```python
from build123d import *

# Parameters (mm, degrees)
SKETCH1_W            = 32
SKETCH1_H            = 26.941935484
SKETCH1_R            = 4
BOSS_EXTRUDE1_DEPTH  = 10
SKETCH2_W            = 10
SKETCH2_H            = 26.941935484
BOSS_EXTRUDE2_DEPTH  = 8
BOSS_EXTRUDE3_REACH  = 61.413
M5_CLEARANCE_HOLE1_D = 5.8
SKETCH6_W            = 52
SKETCH6_H            = 44.941935484
SKETCH6_R            = 4
BOSS_EXTRUDE4_DEPTH  = 6
M5_CLEARANCE_HOLE2_D = 5.8


with BuildPart() as part:
    # Sketch1 → Boss-Extrude1 (new body)
    with BuildSketch(Plane(origin=(0, 0, 0), x_dir=(1, 0, 0), z_dir=(0, 1, 0))):
        with Locations((16, 13.470967742)):
            Rectangle(SKETCH1_W, SKETCH1_H)
        with Locations(Location((16, 13.7, 0), (0, 0, 270))):
            Circle(SKETCH1_R, mode=Mode.SUBTRACT)
    extrude(amount=BOSS_EXTRUDE1_DEPTH)

    # Sketch2 → Boss-Extrude2 (add)
    with BuildSketch(Plane(origin=(0, 10, 0), x_dir=(1, 0, 0), z_dir=(0, 1, 0))):
        with Locations((-5, 13.470967742)):
            Rectangle(SKETCH2_W, SKETCH2_H)
        with Locations((37, 13.470967742)):
            Rectangle(SKETCH2_W, SKETCH2_H)
    extrude(amount=-BOSS_EXTRUDE2_DEPTH)

    # Boss-Extrude3: up to this face of the body (flat: up to its plane)
    boss_extrude3_end = Plane(part.part.faces().sort_by_distance((42, 6, -13.470967742))[0])
    # Sketch3 → Boss-Extrude3 (add, up to the picked face)
    with BuildSketch(Plane.ZY.offset(10), mode=Mode.PRIVATE) as boss_extrude3_sk1:
        Polygon((0, 0), (8, -8), (18, -8), (18, 10), (0, 10), align=None)
    boss_extrude3_tool1 = split(extrude(boss_extrude3_sk1.sketch, amount=-BOSS_EXTRUDE3_REACH, mode=Mode.PRIVATE), bisect_by=boss_extrude3_end, keep=Keep.BOTH, mode=Mode.PRIVATE)
    add(boss_extrude3_tool1.solids().sort_by(Axis((-10, 1.694064, 9.694064), (1, 0, 0)))[0])

    # M5 Clearance Hole1 (through all)
    with Locations(Plane(origin=(0, 0, -26.941935484), x_dir=(-1, 0, 0), z_dir=(0, 0, -1))):
        with Locations((-28, 6), (-4, 6)):
            Hole(M5_CLEARANCE_HOLE1_D / 2)

    # Sketch6 → Boss-Extrude4 (add)
    with BuildSketch(Plane(origin=(0, 10, 0), x_dir=(1, 0, 0), z_dir=(0, 1, 0))):
        with Locations((16, 4.470967742)):
            Rectangle(SKETCH6_W, SKETCH6_H)
        with Locations(Location((16, 13.7, 0), (0, 0, 270))):
            Circle(SKETCH6_R, mode=Mode.SUBTRACT)
    extrude(amount=BOSS_EXTRUDE4_DEPTH)

    # M5 Clearance Hole2 (through all)
    with Locations(Plane(origin=(0, 16, 0), x_dir=(1, 0, 0), z_dir=(0, 1, 0))):
        with Locations((37.04456925, 18.051391355), (36.92194463, 5.790370874), (-4.953330413, 18.47141973), (-5.075955034, 6.210399249)):
            Hole(M5_CLEARANCE_HOLE2_D / 2)


solid = part.part
```
Can you work these out from the model? Positions are in its coordinate system, mm. A direction names the side the tool comes from. Give positions to 0.01 mm unless a question says otherwise; leave off trailing zeros. Write each loop counter-clockwise with the first axis right and the second up, starting at its lowest first coordinate (ties: lowest second). Pieces come first, ordered by that corner, then holes. Notation, with made-up numbers: (-23.5, 72) - (-16.5, 72) arc R26 cw to (-16.5, 109) - close; hole circle Ø7 at (-16, 40). An arc over 180 degrees is marked (long way). Write item = value, one per line. Start each with the question number.
1. Imagine slicing it at B-B (z = -13.7). Please give me the cut outline in (x, y), and give its area (3 significant figures).
2. Imagine slicing it at D-D (y = 6). Please give me the cut outline in (x, z), and give its area (3 significant figures).
3. On a 3-axis mill with a long thin cutter (end or side, diameter ignored), from which of +Z, -Z, +X, -X, +Y, -Y can I reach the whole of each face in a straight line? I mean faces 1 (the face through (19.3, 0, -10.7)), 2 (the face through (32, 1, -13)), 3 (the face through (0, 1, -13)). Say none if no direction works.
4. For pin 1 (13.5 mm diameter, centred on x = 20, z = -14.5, fed in from -Y); pin 2 (1.6 mm diameter, centred on x = 38.5, y = 1, fed in from -Z); pin 3 (3.5 mm diameter, centred on x = 4, y = 6, fed in from -Z); pin 4 (0.6 mm diameter, centred on y = 1, z = -14.5, fed in from -X), each with a flat end and sliding along its axis, tell me the tip position at first contact or that it passes through.
5. Thinking about a two-plate mould opening in Z: for faces 4 (the face through (37, 1, 0)), 5 (the face through (37, 2, -14)), 6 (the face through (-2.65, 8.9, -16.71)), which applies, released by +Z, released by -Z, zero draft, split by the parting line, or undercut?
6. Imagine slicing it at C-C (x = 28). Please give me the cut outline in (y, z), and give its area (3 significant figures).
7. Please list where these lines run through material, in increasing order: line 1 (X direction, y = 4.75, z = -2); line 2 (Z direction, x = 36, y = 13); line 3 (Y direction, x = 4, z = -15.5).
8. Imagine slicing it at A-A (y = 0.75). Please give me the cut outline in (x, z), and give its area (3 significant figures).
Worked answers:
q1.outline = (-10, 2) - (0, 2) - (0, 0) - (12, 0) - (12, 16) - (-10, 16) - close; (20, 0) - (32, 0) - (32, 2) - (42, 2) - (42, 16) - (20, 16) - close; hole circle Ø5.8 at (4, 6); hole circle Ø5.8 at (28, 6)
q1.area = 611 mm2
q2.outline = (-10, -26.94) - (1.1, -26.94) - (1.1, 18) - (-10, 18) - close; (6.9, -26.94) - (25.1, -26.94) - (25.1, 18) - (6.9, 18) - close; (30.9, -26.94) - (42, -26.94) - (42, 18) - (30.9, 18) - close; hole circle Ø5.8 at (-5.08, -6.21); hole circle Ø5.8 at (-4.95, -18.47); hole circle Ø8 at (16, -13.7); hole circle Ø5.8 at (36.92, -5.79); hole circle Ø5.8 at (37.04, -18.05)
q2.area = 1,660 mm2
q3.face_1 = -Z, +X, -X, -Y
q3.face_2 = -Z, +X, -Y
q3.face_3 = -Z, -X, -Y
q4.pin_1 = 0
q4.pin_2 = 0
q4.pin_3 = through
q4.pin_4 = 0
q5.face_4 = released by -Z
q5.face_5 = zero draft
q5.face_6 = undercut
q6.outline = (-8, 8) - (0, 0) - (0, -26.94) - (3.1, -26.94) - (3.1, 18) - (-8, 18) - close; (8.9, -26.94) - (16, -26.94) - (16, 18) - (8.9, 18) - close
q6.area = 570 mm2
q7.line_1 = -10 to 1.38, 6.62 to 25.38, 30.62 to 42
q7.line_2 = -26.94 to -20.76, -15.35 to -8.54, -3.04 to 18
q7.line_3 = 0 to 3.1, 8.9 to 16
q8.outline = (-10, 0) - (0, 0) - (0, -26.94) - (32, -26.94) - (32, 0) - (42, 0) - (42, 18) - (-10, 18) - close; hole circle Ø8 at (16, -13.7)
q8.area = 1,750 mm2
